```python
from build123d import *

# Parameters (mm, degrees)
SKETCH1_R           = 14.859
SKETCH1_R_2         = 4.318
BOSS_EXTRUDE1_DEPTH = 6.604
SKETCH2_R           = 16.51
SKETCH2_R_2         = 4.318
BOSS_EXTRUDE2_DEPTH = 1.27
SKETCH3_R           = 12.7
CUT_EXTRUDE1_DEPTH  = 5.969


with BuildPart() as part:
    # Sketch1 → Boss-Extrude1 (new body)
    with BuildSketch(Plane(origin=(0, 0, 0), x_dir=(1, 0, 0), z_dir=(0, 1, 0))):
        Circle(SKETCH1_R)
        Circle(SKETCH1_R_2, mode=Mode.SUBTRACT)
    extrude(amount=BOSS_EXTRUDE1_DEPTH)

    # Sketch2 → Boss-Extrude2 (add)
    with BuildSketch(Plane(origin=(0, 6.604, 0), x_dir=(1, 0, 0), z_dir=(0, 1, 0))):
        Circle(SKETCH2_R)
        Circle(SKETCH2_R_2, mode=Mode.SUBTRACT)
    extrude(amount=BOSS_EXTRUDE2_DEPTH)

    # Sketch3 → Cut-Extrude1 (cut)
    with BuildSketch(Plane(origin=(0, 7.874, 0), x_dir=(1, 0, 0), z_dir=(0, 1, 0))):
        Circle(SKETCH3_R)
    extrude(amount=-CUT_EXTRUDE1_DEPTH, mode=Mode.SUBTRACT)


solid = part.part
```
The model under review builds one solid part; all positions refer to its coordinate system, in mm. A direction names the side the tool comes from. Give positions to 0.01 mm unless a question says otherwise; leave off trailing zeros. Write each loop counter-clockwise with the first axis right and the second up, starting at its lowest first coordinate (ties: lowest second). Pieces come first, ordered by that corner, then holes. Notation, with made-up numbers: M -21,69 L 9,69 A12 cw 9,76 Z; hole C 62.25,54.25 d4. An arc over 180 degrees is marked long. Write item = value, one per line. Start each with the question number.
Q1. We need section D-D (z = -12). State the section outline as (x, y) points (3 decimals).
Q2. Mouldability with a two-part tool opening along Z and no side actions: class faces 3 (the face through (5, 1.905, 0)), 4 (the face through (15.748, 7.23, -4.959)), 5 (the face through (8.5, 7.874, 9.7)), 6 (the face through (-2.75, 4.93, 12.4)) as released by +Z, released by -Z, zero draft, split by the parting line, or undercut.
Q3. Clearance check with flat-ended pins moving along their axes: pin 1 (2 mm diameter, centred on x = -11.5, y = 1.5, fed in from +Z); pin 2 (3 mm diameter, centred on y = 4, z = 2, fed in from -X); pin 3 (4 mm diameter, centred on y = 5, z = -12, fed in from -X). State where each tip first meets the part, or that it passes through.
Q4. We need section A-A (x = 0). State the section outline as (y, z) points (3 decimals).
Q5. For line 1 (Z direction, x = 0, y = 6.5); line 2 (Z direction, x = 0, y = 1), list the stretches that pass through material, from the lowest coordinate up.
Q6. We need section B-B (z = 0). State the section outline as (x, y) points (3 decimals).
Q7. We need section C-C (y = 5.25). State the section outline as (x, z) points, plus the area to 3 significant figures.
Q8. Machinability: for faces 1 (the face through (-3.221, 3.256, 14.506)), 2 (the face through (3, 0, -4)), which of the approach directions +Z, -Z, +X, -X, +Y, -Y give a long, thin tool a straight path to every point of the face, cutting with its end or side? Answer none if there is none.
Result set:
q1.outline = M -11.339,6.604 L -8.763,6.604 L -8.763,0 L 8.763,0 L 8.763,6.604 L 11.339,6.604 L 11.339,7.874 L 4.158,7.874 L 4.158,1.905 L -4.158,1.905 L -4.158,7.874 L -11.339,7.874 Z
q2.face_3 = undercut
q2.face_4 = split by the parting line
q2.face_5 = zero draft
q2.face_6 = undercut
q3.pin_1 = 10.51
q3.pin_2 = -14.85
q3.pin_3 = -12.48
q4.outline = M 0,-14.859 L 6.604,-14.859 L 6.604,-16.51 L 7.874,-16.51 L 7.874,-12.7 L 1.905,-12.7 L 1.905,-4.318 L 0,-4.318 Z; M 0,4.318 L 1.905,4.318 L 1.905,12.7 L 7.874,12.7 L 7.874,16.51 L 6.604,16.51 L 6.604,14.859 L 0,14.859 Z
q5.line_1 = -14.86 to -12.7, 12.7 to 14.86
q5.line_2 = -14.86 to -4.32, 4.32 to 14.86
q6.outline = M -16.51,6.604 L -14.859,6.604 L -14.859,0 L -4.318,0 L -4.318,1.905 L -12.7,1.905 L -12.7,7.874 L -16.51,7.874 Z; M 4.318,0 L 14.859,0 L 14.859,6.604 L 16.51,6.604 L 16.51,7.874 L 12.7,7.874 L 12.7,1.905 L 4.318,1.905 Z
q7.outline = C 0,0 d29.72; hole C 0,0 d25.4
q7.area = 187 mm2
q8.face_1 = -Y
q8.face_2 = +Z, -Z, +X, -X, -Y
